Geometry: final body of the model. Coordinates: model frame, mm. Face numbers are marked on the shaded views. A direction names the side the tool comes from. Give positions to 0.01 mm unless a question says otherwise; leave off trailing zeros. Write each loop counter-clockwise with the first axis right and the second up, starting at its lowest first coordinate (ties: lowest second). Pieces come first, ordered by that corner, then holes.
Q1. Pin query (flat end, axial travel): pin 1 Ø6.5 at (x, y) = (-1, -1) entering from +Z; pin 2 Ø1 at (x, y) = (3, 3.5) entering from +Z; pin 3 Ø8 at (y, z) = (-6.5, 13.5) entering from +X. Return the tip coordinate at first contact, or that it passes through.
Q2. Reachability of the marked faces 1, 2 and 3 from +Z, -Z, +X, -X, +Y, -Y: full face, straight path, thin tool, end or side. Return the list, or none.
Q3. Section B-B (y = -5). Return the cut outline in (x, z).
Q4. Line query: line 1 (Y direction, x = 0.75, z = 11.5); line 2 (Y direction, x = -8.5, z = 14.25); line 3 (X direction, y = -6, z = 9.25). Output: solid intervals per line, ascending.
Q5. Section A-A (z = 7.5). Return the cut outline in (x, y).
Q6. Section D-D (y = 8.25). Return the cut outline in (x, z).
Q7. Section C-C (z = 11). Return the cut outline in (x, y), plus the area to 3 significant figures.
Q8. Mould query, pull axis Y, two halves, no side actions, for the marked faces 4, 5 and 6. Classes: +Y half, -Y half, draft (parallel to the pull), parting line (faces both ways), or undercut.
from build123d import *

# Parameters (mm, degrees)
SKETCH1_W               = 20
SKETCH1_H               = 18
BOSS_EXTRUDE1_DEPTH     = 7
SKETCH2_W               = 20
SKETCH2_H               = 6
BOSS_EXTRUDE2_DEPTH     = 15
CUT_EXTRUDE1_REACH      = 32.133
SKETCH3_R               = 5.35
SKETCH5_W               = 14
SKETCH5_H               = 6
CUT_EXTRUDE2_DEPTH      = 26.787593916
FILLET1_R               = 0.3
SKETCH6_W               = 20
SKETCH6_H               = 9
CUT_EXTRUDE3_DEPTH      = 21.149441799
CUT_EXTRUDE3_DEPTH_BACK = 21.149441799
SKETCH7_R               = 2
CUT_EXTRUDE4_DEPTH      = 26.787594037
CUT_EXTRUDE4_DEPTH_BACK = 26.787594037


with BuildPart() as part:
    # Sketch1 → Boss-Extrude1 (new body)
    with BuildSketch(Plane.XY):
        Rectangle(SKETCH1_W, SKETCH1_H)
    extrude(amount=BOSS_EXTRUDE1_DEPTH)

    # Sketch2 → Boss-Extrude2 (add)
    with BuildSketch(Plane.XY.offset(7)):
        with Locations((0, -6)):
            Rectangle(SKETCH2_W, SKETCH2_H)
        with Locations((0, 6)):
            Rectangle(SKETCH2_W, SKETCH2_H)
    extrude(amount=BOSS_EXTRUDE2_DEPTH)

    # Cut-Extrude1: up to this face of the body (flat: up to its plane)
    cut_extrude1_end = Plane(part.part.faces().sort_by_distance((0, 9, 11))[0])
    # Sketch3 → Cut-Extrude1 (cut, up to the picked face)
    with BuildSketch(Plane.XZ.offset(9), mode=Mode.PRIVATE) as cut_extrude1_sk1:
        with Locations((0, 19.5)):
            Circle(SKETCH3_R)
    cut_extrude1_tool1 = split(extrude(cut_extrude1_sk1.sketch, amount=-CUT_EXTRUDE1_REACH, mode=Mode.PRIVATE), bisect_by=cut_extrude1_end, keep=Keep.BOTH, mode=Mode.PRIVATE)
    # Sketch3 → Cut-Extrude1 (cut, up to the picked face)
    with BuildSketch(Plane.XZ.offset(9), mode=Mode.PRIVATE) as cut_extrude1_sk2:
        Polygon((-7, 22), (-10, 7), (-10, 22), align=None)
    cut_extrude1_tool2 = split(extrude(cut_extrude1_sk2.sketch, amount=-CUT_EXTRUDE1_REACH, mode=Mode.PRIVATE), bisect_by=cut_extrude1_end, keep=Keep.BOTH, mode=Mode.PRIVATE)
    # Sketch3 → Cut-Extrude1 (cut, up to the picked face)
    with BuildSketch(Plane.XZ.offset(9), mode=Mode.PRIVATE) as cut_extrude1_sk3:
        Polygon((7, 22), (10, 22), (10, 7), align=None)
    cut_extrude1_tool3 = split(extrude(cut_extrude1_sk3.sketch, amount=-CUT_EXTRUDE1_REACH, mode=Mode.PRIVATE), bisect_by=cut_extrude1_end, keep=Keep.BOTH, mode=Mode.PRIVATE)
    add(cut_extrude1_tool1.solids().sort_by(Axis((0, -9, 19.5), (0, 1, 0)))[0], mode=Mode.SUBTRACT)
    add(cut_extrude1_tool2.solids().sort_by(Axis((-9, -9, 17), (0, 1, 0)))[0], mode=Mode.SUBTRACT)
    add(cut_extrude1_tool3.solids().sort_by(Axis((9, -9, 17), (0, 1, 0)))[0], mode=Mode.SUBTRACT)

    # Sketch4 → Revolve4 (revolve)
    with BuildSketch(Plane.XY.offset(19.5), mode=Mode.PRIVATE) as revolve4_sk:
        with BuildLine():
            Line((-4.781378582, -5.843107092), (-5.35, -3))
            Line((-5.35, -3), (-5.35, -6))
            Line((-5.35, -6), (-4.765843122, -6))
            ThreePointArc((-4.765843122, -6), (-4.769736461, -5.921169906), (-4.781378582, -5.843107092))
        make_face()
        with BuildLine():
            Line((-4.765843122, -6), (-5.35, -6))
            Line((-5.35, -6), (-5.35, -9))
            Line((-5.35, -9), (-4.781378582, -6.156892908))
            ThreePointArc((-4.781378582, -6.156892908), (-4.769736461, -6.078830094), (-4.765843122, -6))
        make_face()
    revolve(revolve4_sk.sketch.rotate(Axis((0, -3, 19.5), (0, -1, 0)), 270), axis=Axis((0, -3, 19.5), (0, -1, 0)))

    # Sketch5 → Cut-Extrude2 (cut, through all)
    with BuildSketch(Plane.XY.offset(22)):
        with Locations((0, -6)):
            Rectangle(SKETCH5_W, SKETCH5_H)
    extrude(amount=CUT_EXTRUDE2_DEPTH, mode=Mode.SUBTRACT)

    # Fillet1
    fillet1_edges = [part.edges().sort_by_distance(p)[0] for p in [
        (7, -6, 22),
        (-7, -6, 22),
        (-7, 6, 22),
        (7, 6, 22),
        (-4.729957717, 6, 22),
        (4.729957717, 6, 22),
    ]]
    fillet(fillet1_edges, radius=FILLET1_R)

    # Sketch6 → Cut-Extrude3 (cut, two sides)
    with BuildSketch(Plane.XY.offset(7)) as cut_extrude3_sk:
        with Locations((0, 4.5)):
            Rectangle(SKETCH6_W, SKETCH6_H)
    extrude(amount=CUT_EXTRUDE3_DEPTH, mode=Mode.SUBTRACT)
    extrude(cut_extrude3_sk.sketch, amount=-CUT_EXTRUDE3_DEPTH_BACK, mode=Mode.SUBTRACT)

    # Mirror2: part across plane


with BuildPart() as part_1:
    add(part.part)
    add(part.part.mirror(Plane(origin=(-10, 0, 0), x_dir=(0, 0, 1), z_dir=(0, -1, 0))))

    # Sketch7 → Cut-Extrude4 (cut, two sides)
    with BuildSketch(Plane(origin=(0, 0, 0), x_dir=(-1, 0, 0), z_dir=(0, 0, -1))) as cut_extrude4_sk:
        with Locations((0, -6)):
            Circle(SKETCH7_R)
    extrude(amount=CUT_EXTRUDE4_DEPTH, mode=Mode.SUBTRACT)
    extrude(cut_extrude4_sk.sketch, amount=-CUT_EXTRUDE4_DEPTH_BACK, mode=Mode.SUBTRACT)

    # Sketch8 → Cut-Revolve1 (revolve, cut)
    with BuildSketch(Plane.XY.offset(19.5)):
        with BuildLine():
            Line((-6.116799524, -6.580040554), (-5.065689291, -7.578446454))
            Line((-5.065689291, -7.578446454), (-4.781378582, -6.156892908))
            ThreePointArc((-4.781378582, -6.156892908), (-4.765843122, -6), (-4.781378582, -5.843107092))
            Line((-4.781378582, -5.843107092), (-5.065689291, -4.421553546))
            Line((-5.065689291, -4.421553546), (-6.116799524, -5.419959446))
            ThreePointArc((-6.116799524, -5.419959446), (-6.365843122, -6), (-6.116799524, -6.580040554))
        make_face()
    revolve(axis=Axis((0, -3, 19.5), (0, -1, 0)), mode=Mode.SUBTRACT)


solid = part_1.part
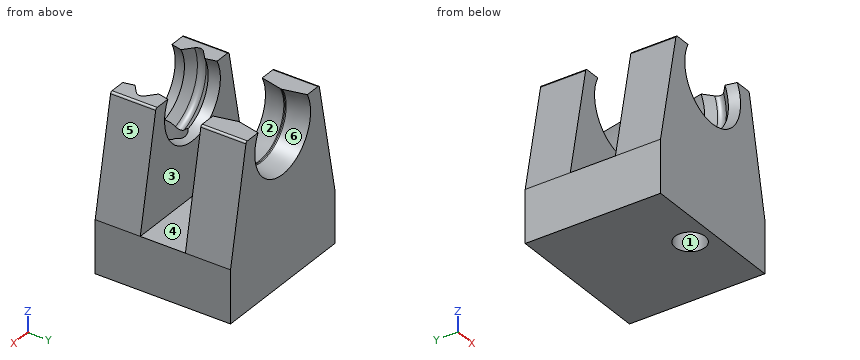
Computed:
1. pin 1: stops at z = 15.51
1. pin 2: stops at z = 15.61
1. pin 3: stops at x = 9.5
2. face 1: +Z, -Z
2. face 2: none
2. face 3: +Z, +X, -X
3. outline: (-10, 0) - (-1.73, 0) - (-1.73, 14.1) arc R5.67 cw to (-5.09, 22) - (-6.75, 22) arc R0.3 ccw to (-7.05, 21.76) - (-10, 7) - close; (1.73, 0) - (10, 0) - (10, 7) - (7.05, 21.76) arc R0.3 ccw to (6.75, 22) - (5.09, 22) arc R5.67 cw to (1.73, 14.1) - close
4. line 1: y = -9 to -7.85, -4.15 to -3, 3 to 9
4. line 2: y = -9 to -3, 3 to 9
4. line 3: x = -9.55 to -2, 2 to 9.55
5. outline: (-9.9, -9) - (9.9, -9) - (9.9, -3) - (-9.9, -3) - close; (-9.9, 3) - (9.9, 3) - (9.9, 9) - (-9.9, 9) - close; hole circle Ø4 at (0, -6)
6. outline: (-10, 0) - (10, 0) - (10, 7) - (7.05, 21.76) arc R0.3 ccw to (6.75, 22) - (4.56, 22) arc R5.2 cw (long way) to (-4.56, 22) - (-6.75, 22) arc R0.3 ccw to (-7.05, 21.76) - (-10, 7) - close
7. outline: (-9.2, -9) - (9.2, -9) - (9.2, -3) - (-9.2, -3) - close; (-9.2, 3) - (9.2, 3) - (9.2, 9) - (-9.2, 9) - close; hole circle Ø4 at (0, -6)
7. area: 208 mm2
8. face 4: undercut
8. face 5: draft
8. face 6: +Y half
